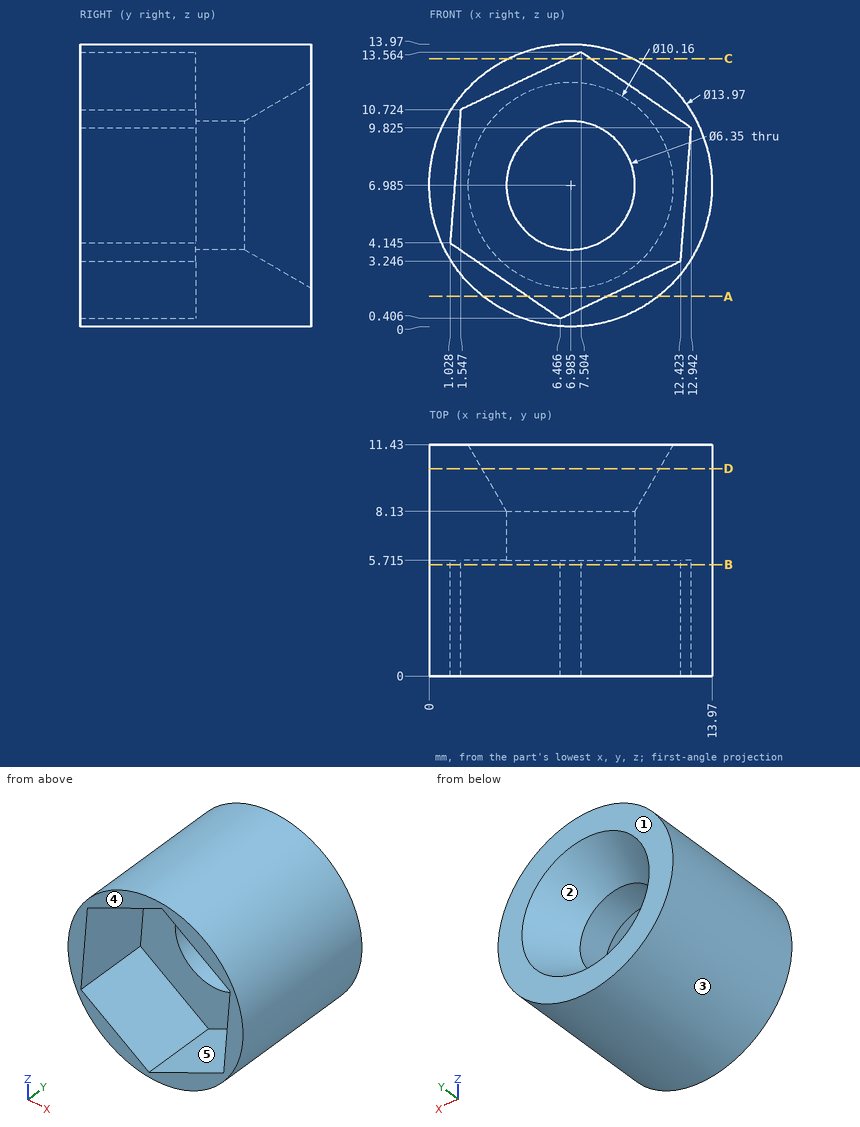
The figure shows three views and two pictorial views of one solid part (mm, origin at its lowest corner). Answer the questions. A direction names the side the tool comes from. Give positions to 0.01 mm unless a question says otherwise; leave off trailing zeros. Order: outer loops, then holes, each group sorted by start corner. A loop starts at its lowest first (then second) coordinate and runs counter-clockwise, first axis right, second up. Notation, with made-up numbers: M 68.5,7.5 L 126.5,7.5 A16 cw 126.5,33.5 Z; hole C 84,36 d6. An arc over 180 degrees is marked long. Return JSON: item names as keys, results as strings.
Q1. Find the intervals of material crossed by line 1 along X through (y, z) = (10, 9) (1 decimal); line 2 along X through (y, z) = (5.25, 6.5) (1 decimal); line 3 along Y through (x, z) = (2.75, 10) (1 decimal), in increasing order. Write a range as [from, to].
Answer below:
{"line 1": "x = [0.3, 3.2], [10.7, 13.7]", "line 2": "x = [0, 1.2], [12.7, 14]", "line 3": "y = [5.7, 11.4]"}
Q2. Each of these flat-tipped pins is pushed along its axis until it touches: pin 1 (4 mm diameter, centred on x = 2, y = 5, fed in from +Z); pin 2 (1 mm diameter, centred on y = 10, z = 2.5, fed in from -X); pin 3 (3 mm diameter, centred on y = 9.5, z = 3, fed in from -X). Where does it stop, or does it pass through?
Answer below:
{"pin 1": "stops at z = 13.3", "pin 2": "stops at x = 1.25", "pin 3": "stops at x = 0.46"}
Q3. Find section B-B, the plane y = 5.5. Write down the section's boundary in (x, z) (1 decimal).
Answer below:
{"outline": "C 7,7 d14; hole M 1,4.1 L 6.5,0.4 L 12.4,3.2 L 12.9,9.8 L 7.5,13.6 L 1.5,10.7 Z"}
Q4. Which of the six approach directions +Z, -Z, +X, -X, +Y, -Y give full straight-line access (tool end or side, diameter ignored) to the marked faces 4 and 5?
Answer below:
{"face 4": "+Z, -Z, +X, -X, -Y", "face 5": "-Y"}
Q5. Find section A-A, the plane z = 1.5. Write down the section's boundary in (x, y) (1 decimal).
Answer below:
{"outline": "M 2.7,0 L 4.9,0 L 4.9,5.7 L 8.8,5.7 L 8.8,0 L 11.3,0 L 11.3,11.4 L 2.7,11.4 Z"}
Q6. Find section C-C, the plane z = 13.25. Write down the section's boundary in (x, y) (1 decimal).
Answer below:
{"outline": "M 3.9,0 L 6.8,0 L 6.8,5.7 L 8,5.7 L 8,0 L 10.1,0 L 10.1,11.4 L 3.9,11.4 Z"}
Q7. The mould has two halves that part along Z. Classify the marked faces 1, 2 and 3: pulls with the +Z half, pulls with the -Z half, needs draft (parallel to the pull), parting line crosses it, or undercut.
Answer below:
{"face 1": "needs draft", "face 2": "undercut", "face 3": "parting line crosses it"}
Q8. Find section D-D, the plane y = 10.25. Write down the section's boundary in (x, z) (1 decimal).
Answer below:
{"outline": "C 7,7 d14; hole C 7,7 d8.8"}
